Can you work these out from the model? Positions are in its coordinate system, mm. Give positions to 0.01 mm unless a question says otherwise; leave off trailing zeros. Order: outer loops, then holes, each group sorted by start corner. A loop starts at its lowest first (then second) coordinate and runs counter-clockwise, first axis right, second up. Notation, with made-up numbers: (-30, 24) -> (-16, 24) arc R25 cw to (-16, 48) -> close; hole circle Ø10 at (-9, 49.25). An arc over 180 degrees is marked (long way). Answer as CSV lines item,"result".
```python
from build123d import *

# Parameters (mm, degrees)
SKETCH1_R               = 82
BOSS_EXTRUDE1_DEPTH     = 4
SKETCH2_R               = 2
CUT_EXTRUDE1_DEPTH      = 8
CIRPATTERN1_COUNT       = 2
CUT_EXTRUDE2_DEPTH      = 117.034477635
CUT_EXTRUDE2_DEPTH_BACK = 10


with BuildPart() as part:
    # Sketch1 → Boss-Extrude1 (new body)
    with BuildSketch(Plane.XY):
        Circle(SKETCH1_R)
    extrude(amount=BOSS_EXTRUDE1_DEPTH)

    # Sketch2 → Cut-Extrude1 (cut)
    with BuildSketch(Plane.XY.offset(4)):
        with Locations((0, 60)):
            Circle(SKETCH2_R)
    cut_extrude1 = extrude(amount=-CUT_EXTRUDE1_DEPTH, mode=Mode.SUBTRACT)

    # CirPattern1: Cut-Extrude1 ×2 about axis
    cirpattern1_axis = Axis((0, 0, 0), (0, 0, 1))
    for i in range(1, CIRPATTERN1_COUNT):
        add(cut_extrude1.rotate(cirpattern1_axis, i * 360 / CIRPATTERN1_COUNT), mode=Mode.SUBTRACT)

    # Sketch3 → Cut-Extrude2 (cut, two sides: drawn at the far end of the back side and taken through both)
    with BuildSketch(Plane.XY.offset(4).offset(-CUT_EXTRUDE2_DEPTH_BACK)):
        with BuildLine():
            ThreePointArc((-61.479450169, 54.261194301), (-82, 0), (-61.479450169, -54.261194301))
            Line((-61.479450169, -54.261194301), (-61.479450169, 54.261194301))
        make_face()
        with BuildLine():
            Line((61.479450169, 54.261194301), (61.479450169, 31.325344482))
            ThreePointArc((61.479450169, 31.325344482), (67.093524507, 16.107730106), (69, 0))
            Line((69, 0), (82, 0))
            ThreePointArc((82, 0), (76.698484059, 29.005905314), (61.479450169, 54.261194301))
        make_face()
        with BuildLine():
            Line((61.479450169, 0), (61.479450169, -31.325344482))
            ThreePointArc((61.479450169, -31.325344482), (67.093524507, -16.107730106), (69, 0))
            Line((69, 0), (61.479450169, 0))
        make_face()
        with BuildLine():
            ThreePointArc((69, 0), (67.093524507, 16.107730106), (61.479450169, 31.325344482))
            Line((61.479450169, 31.325344482), (61.479450169, 0))
            Line((61.479450169, 0), (69, 0))
        make_face()
        with BuildLine():
            ThreePointArc((69, 0), (67.093524507, -16.107730106), (61.479450169, -31.325344482))
            Line((61.479450169, -31.325344482), (73.062534983, -37.227220979))
            ThreePointArc((73.062534983, -37.227220979), (79.734333473, -19.142519836), (82, 0))
            Line((82, 0), (69, 0))
        make_face()
        with BuildLine():
            Line((73.062534983, -37.227220979), (61.479450169, -31.325344482))
            Line((61.479450169, -31.325344482), (61.479450169, -54.261194301))
            ThreePointArc((61.479450169, -54.261194301), (67.808004719, -46.109375359), (73.062534983, -37.227220979))
        make_face()
    extrude(amount=CUT_EXTRUDE2_DEPTH + CUT_EXTRUDE2_DEPTH_BACK, mode=Mode.SUBTRACT)


solid = part.part
```
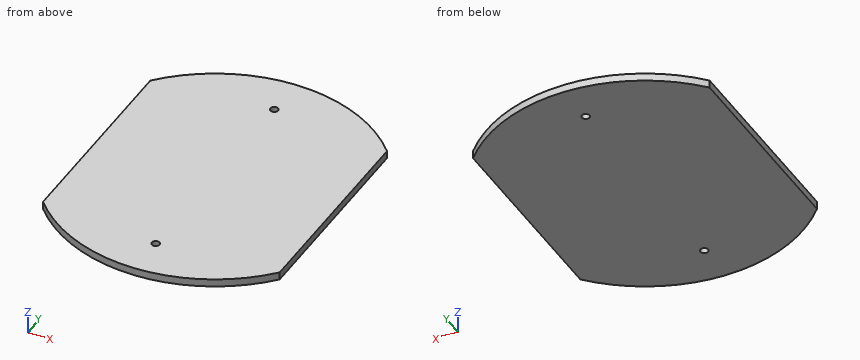
Item 1: Imagine slicing it at A-A, the plane x = 0. Please give me the cut outline in (y, z).
Numbers:
outline,"(-82, 0) -> (-62, 0) -> (-62, 4) -> (-82, 4) -> close; (-58, 0) -> (58, 0) -> (58, 4) -> (-58, 4) -> close; (62, 0) -> (82, 0) -> (82, 4) -> (62, 4) -> close"
Item 2: Please list where these lines run through material, in increasing order: line 1 along Y through (x, z) = (0, 2.9); line 2 along X through (y, z) = (-60, 1.25); line 3 along Y through (x, z) = (-55, 1.05).
Numbers:
line 1,"y = -82 to -62, -58 to 58, 62 to 82"
line 2,"x = -55.89 to -2, 2 to 55.89"
line 3,"y = -60.82 to 60.82"
Item 3: Imagine slicing it at C-C, the plane z = 3.15. Please give me the cut outline in (x, y).
Numbers:
outline,"(-61.48, -54.26) arc R82 ccw to (61.48, -54.26) -> (61.48, 54.26) arc R82 ccw to (-61.48, 54.26) -> close; hole circle Ø4 at (0, -60); hole circle Ø4 at (0, 60)"
Item 4: Imagine slicing it at B-B, the plane y = -60. Please give me the cut outline in (x, z), then the cut area to 3 significant figures.
Numbers:
outline,"(-55.89, 0) -> (-2, 0) -> (-2, 4) -> (-55.89, 4) -> close; (2, 0) -> (55.89, 0) -> (55.89, 4) -> (2, 4) -> close"
area,"431 mm²"
Item 5: For pin 1 (1 mm diameter, centred on x = 6, z = 1.5, fed in from +Y), with a flat end and sliding along its axis, tell me the tip position at first contact or that it passes through.
Numbers:
pin 1,"stops at y = 81.82"
Item 6: Imagine slicing it at D-D, the plane x = -29. Please give me the cut outline in (y, z), then the cut area to 3 significant figures.
Numbers:
outline,"(-76.7, 0) -> (76.7, 0) -> (76.7, 4) -> (-76.7, 4) -> close"
area,"614 mm²"
